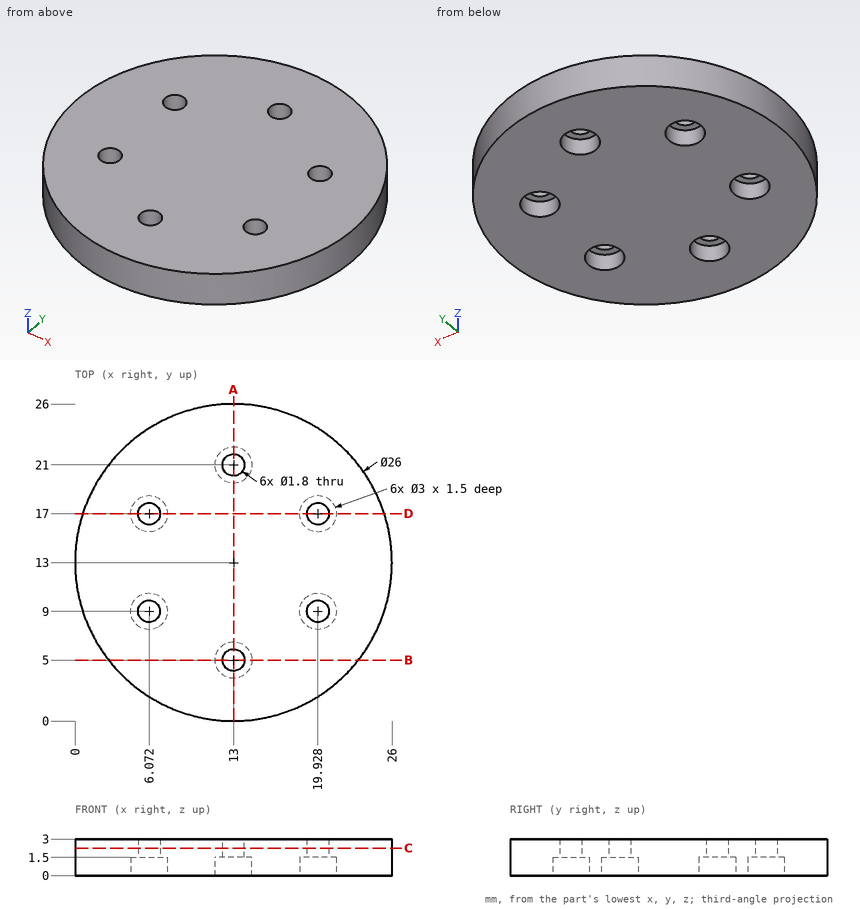
Design review of the part shown in the three views and the two pictorial views. Dimensions are in mm from the part's minimum x, y and z. Round coordinates to 2 decimals unless told otherwise and drop trailing zeros. Write each loop counter-clockwise with the first axis right and the second up, starting at its lowest first coordinate (ties: lowest second). Pieces come first, ordered by that corner, then holes. Notation, with made-up numbers: M 65.25,86 L 97.25,86 A13 ccw 97.25,102 Z; hole C 38,49 d9. An arc over 180 degrees is marked long. Use a Markdown table: item, result. Add a question column.
Q1. We need section C-C, the plane z = 2.25. State the section outline as (x, y) points, plus the area to 3 significant figures.
Q2. We need section D-D, the plane y = 17. State the section outline as (x, z) points.
Q3. To check wall thickness, follow line 1 (Y direction, x = 13, z = 1.1); line 2 (Y direction, x = 13, z = 2.4); line 3 (Y direction, x = 7.5, z = 2.1). State the ranges of each line that lie inside material, in increasing order.
Q4. Insertion check: pin 1 (2.5 mm diameter, centred on x = 20, y = 17, fed in from -Z); pin 2 (1 mm diameter, centred on x = 19, z = 1.5, fed in from +Y); pin 3 (1 mm diameter, centred on y = 12, z = 2, fed in from -X); pin 4 (1.4 mm diameter, centred on x = 19.93, y = 9, fed in from +Z). Each pin has a flat end and moves straight along its axis. Give the tip position at first contact, or say it passes through.
Q5. We need section A-A, the plane x = 13. State the section outline as (y, z) points.
Q6. We need section B-B, the plane y = 5. State the section outline as (x, z) points.
Findings below:
| question | item | result |
|---|---|---|
| 1 | outline | C 13,13 d26; hole C 6.07,9 d1.8; hole C 6.07,17 d1.8; hole C 13,5 d1.8; hole C 13,21 d1.8; hole C 19.93,9 d1.8; hole C 19.93,17 d1.8 |
| 1 | area | 516 mm² |
| 2 | outline | M 0.63,0 L 4.57,0 L 4.57,1.5 L 5.17,1.5 L 5.17,3 L 0.63,3 Z; M 6.97,1.5 L 7.57,1.5 L 7.57,0 L 18.43,0 L 18.43,1.5 L 19.03,1.5 L 19.03,3 L 6.97,3 Z; M 20.83,1.5 L 21.43,1.5 L 21.43,0 L 25.37,0 L 25.37,3 L 20.83,3 Z |
| 3 | line 1 | y = 0 to 3.5, 6.5 to 19.5, 22.5 to 26 |
| 3 | line 2 | y = 0 to 4.1, 5.9 to 20.1, 21.9 to 26 |
| 3 | line 3 | y = 1.22 to 24.78 |
| 4 | pin 1 | stops at z = 1.5 |
| 4 | pin 2 | stops at y = 24.78 |
| 4 | pin 3 | stops at x = 0.01 |
| 4 | pin 4 | passes through |
| 5 | outline | M 0,0 L 3.5,0 L 3.5,1.5 L 4.1,1.5 L 4.1,3 L 0,3 Z; M 5.9,1.5 L 6.5,1.5 L 6.5,0 L 19.5,0 L 19.5,1.5 L 20.1,1.5 L 20.1,3 L 5.9,3 Z; M 21.9,1.5 L 22.5,1.5 L 22.5,0 L 26,0 L 26,3 L 21.9,3 Z |
| 6 | outline | M 2.75,0 L 11.5,0 L 11.5,1.5 L 12.1,1.5 L 12.1,3 L 2.75,3 Z; M 13.9,1.5 L 14.5,1.5 L 14.5,0 L 23.25,0 L 23.25,3 L 13.9,3 Z |
